The drawing under review shows one solid part. Ordinate dimensions are in mm from its lowest x, y, z. A direction names the side the tool comes from. Round coordinates to 2 decimals unless told otherwise and drop trailing zeros. Order: outer loops, then holes, each group sorted by start corner. A loop starts at its lowest first (then second) coordinate and runs counter-clockwise, first axis right, second up. Notation, with made-up numbers: M -10.75,19 L -0.75,19 A32 cw -0.75,57 Z; hole C 57,42 d2. An arc over 180 degrees is marked long. Use a Markdown table: item, result.
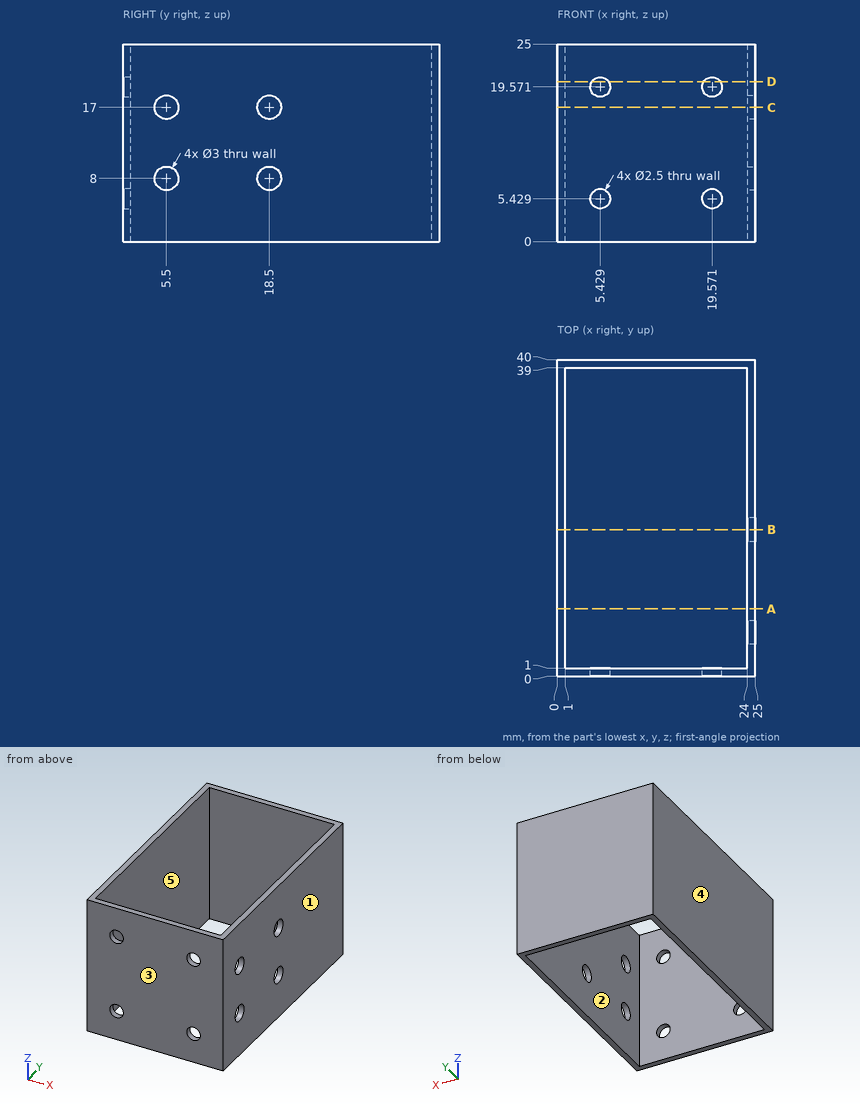
Q1. Add section A-A (y = 8.5). Write out the cut boundary in (x, z).
Determined:
| item | result |
|---|---|
| outline | M 0,0 L 1,0 L 1,25 L 0,25 Z; M 24,0 L 25,0 L 25,25 L 24,25 Z |
Q2. Add section D-D (z = 20.25). Write out the cut boundary in (x, y).
Determined:
| item | result |
|---|---|
| outline | M 0,0 L 4.38,0 L 4.38,1 L 1,1 L 1,39 L 24,39 L 24,1 L 20.62,1 L 20.62,0 L 25,0 L 25,40 L 0,40 Z; M 6.48,0 L 18.52,0 L 18.52,1 L 6.48,1 Z |
Q3. Draft analysis for pull direction Y (two halves, no side actions). For the marked faces 1, 2 and 3, state which applies: pulls with the +Y half, pulls with the -Y half, needs draft (parallel to the pull), parting line crosses it, or undercut.
Determined:
| item | result |
|---|---|
| face 1 | needs draft |
| face 2 | undercut |
| face 3 | pulls with the -Y half |
Q4. Add section C-C (z = 17). Write out the cut boundary in (x, y), then the cut area to 3 significant figures.
Determined:
| item | result |
|---|---|
| outline | M 0,0 L 25,0 L 25,4 L 24,4 L 24,1 L 1,1 L 1,39 L 24,39 L 24,20 L 25,20 L 25,40 L 0,40 Z; M 24,7 L 25,7 L 25,17 L 24,17 Z |
| area | 120 mm^2 |
Q5. Add section B-B (y = 18.5). Write out the cut boundary in (x, z).
Determined:
| item | result |
|---|---|
| outline | M 0,0 L 1,0 L 1,25 L 0,25 Z; M 24,0 L 25,0 L 25,6.5 L 24,6.5 Z; M 24,9.5 L 25,9.5 L 25,15.5 L 24,15.5 Z; M 24,18.5 L 25,18.5 L 25,25 L 24,25 Z |
Q6. Clearance check with flat-ended pins moving along their axes: pin 1 (5 mm diameter, centred on x = 20.5, y = 19, fed in from -Z); pin 2 (2.5 mm diameter, centred on y = 5.5, z = 17, fed in from +X). State where each tip first meets the part, or that it passes through.
Determined:
| item | result |
|---|---|
| pin 1 | passes through |
| pin 2 | stops at x = 1 |
Q7. Machinability: for the marked faces 4 and 5, which of the approach directions +Z, -Z, +X, -X, +Y, -Y give a long, thin tool a straight path to every point of the face, cutting with its end or side? Answer none if there is none.
Determined:
| item | result |
|---|---|
| face 4 | +Z, -Z, -X, +Y, -Y |
| face 5 | +Z, -Z |
Q8. Wall thickness on line 1 along Y through (x, z) = (24.6, 8); line 2 along X through (y, z) = (13, 15); line 3 along Y through (x, z) = (11, 15.5): over which ranges is each line inside the solid? List them lowest first. Write a range as [from, to].
Determined:
| item | result |
|---|---|
| line 1 | y = [0, 4], [7, 17], [20, 40] |
| line 2 | x = [0, 1], [24, 25] |
| line 3 | y = [0, 1], [39, 40] |
